The listing builds one solid part. Answer for the finished solid, in the listing's coordinates (mm). A direction names the side the tool comes from. Give positions to 0.01 mm unless a question says otherwise; leave off trailing zeros. Write each loop counter-clockwise with the first axis right and the second up, starting at its lowest first coordinate (ties: lowest second). Pieces come first, ordered by that corner, then holes.
```python
from build123d import *

# Parameters (mm, degrees)
F0_R     = 10
F1_DEPTH = 2
F2_R     = 4.5
F3_DEPTH = 3.5
F5_R     = 6
F6_DEPTH = 0.5
F7_SIZE  = 0.6


with BuildPart() as f1:
    # F0 (on Front) → F1 (new body)
    with BuildSketch(Plane.XZ):
        Circle(F0_R)
    extrude(amount=F1_DEPTH)

    # F2 (on face) → F3 (join)
    with BuildSketch(Plane.XZ.offset(2)):
        Circle(F2_R)
    extrude(amount=F3_DEPTH)

    # F5 (on face) → F6 (join)
    with BuildSketch(Plane.XZ.offset(2)):
        Circle(F5_R)
    extrude(amount=F6_DEPTH)

    # F7
    f7_edges = [f1.edges().sort_by_distance(p)[0] for p in [
        (-10, 0, 0),
        (-4.5, -5.5, 0),
    ]]
    chamfer(f7_edges, length=F7_SIZE)


solid = f1.part
```
Item 1: A cutting plane is placed at B-B, the plane z = 0. Give the vertices of the cut face in (x, y).
Conclusion:
outline: (-10, -2) - (-6, -2) - (-6, -2.5) - (-4.5, -2.5) - (-4.5, -4.9) - (-3.9, -5.5) - (3.9, -5.5) - (4.5, -4.9) - (4.5, -2.5) - (6, -2.5) - (6, -2) - (10, -2) - (10, -0.6) - (9.4, 0) - (-9.4, 0) - (-10, -0.6) - close
Item 2: Consider probe 1 along Y at (x, z) = (-7, 2); probe 2 along Z at (x, y) = (5, -2.1); probe 3 along X at (y, z) = (-2.45, 0.5). Determine where each line is inside the solid, lowest interval first.
Conclusion:
probe 1: y = -2 to 0
probe 2: z = -3.32 to 3.32
probe 3: x = -5.98 to 5.98
Item 3: Which of the six approach directions +Z, -Z, +X, -X, +Y, -Y give full straight-line access (tool end or side, diameter ignored) to faces 1 (the face through (0, -5.5, 0)), 2 (the face through (0, -2, -7))?
Conclusion:
face 1: +Z, -Z, +X, -X, -Y
face 2: -Y
Item 4: Each of these flat-tipped pins is pushed along its axis until it touches: P1, Ø1.5, axis at y = -3, z = 4, coming from the +X side; P2, Ø1.5, axis at y = -1.5, z = 6, coming from the -X side; P3, Ø1, axis at x = -5.5, z = -6.5, coming from the -Y side. Where does it stop, or does it pass through?
Conclusion:
P1: stops at x = 4.92
P2: stops at x = -8.51
P3: stops at y = -2
Item 5: A cutting plane is placed at C-C, the plane y = -2.8. Give the vertices of the cut face in (x, z).
Conclusion:
outline: circle Ø9 at (0, 0)
Item 6: A cutting plane is placed at A-A, the plane x = 0. Give the vertices of the cut face in (y, z), plus the area to 3 significant figures.
Conclusion:
outline: (-5.5, -3.9) - (-4.9, -4.5) - (-2.5, -4.5) - (-2.5, -6) - (-2, -6) - (-2, -10) - (-0.6, -10) - (0, -9.4) - (0, 9.4) - (-0.6, 10) - (-2, 10) - (-2, 6) - (-2.5, 6) - (-2.5, 4.5) - (-4.9, 4.5) - (-5.5, 3.9) - close
area: 72.3 mm2
Item 7: Determine the mould class of faces 3 (the face through (-1.4, -2.5, 4.5)), 4 (the face through (-0.59, -3.68, 4.46)) for opening direction X: pulls with the +X half, pulls with the -X half, needs draft (parallel to the pull), parting line crosses it, or undercut.
Conclusion:
face 3: needs draft
face 4: parting line crosses it
